Source: CAD feature listing. Evaluate the final solid. Frame: model axes, mm. Round coordinates to 2 decimals unless told otherwise and drop trailing zeros. Write each loop counter-clockwise with the first axis right and the second up, starting at its lowest first coordinate (ties: lowest second). Pieces come first, ordered by that corner, then holes. Notation, with made-up numbers: M 22,29 L 37,29 A21 cw 37,47 Z; hole C 48.25,54 d1. An arc over 180 degrees is marked long. Put each result on its own line as item: value. Start each with the question number.
```python
from build123d import *

# Parameters (mm, degrees)
SCHIZZO1_R                   = 17
SCHIZZO1_R_2                 = 2
SCHIZZO1_R_3                 = 4.5
SCHIZZO1_R_4                 = 1.5
ESTRUSIONE_ESTRUSIONE1_DEPTH = 15
M8_TAPPED_HOLE1_D            = 6.8
M8_TAPPED_HOLE1_DEPTH        = 23.75
M8_TAPPED_HOLE1_TIP          = 2.042926105


with BuildPart() as part:
    # Schizzo1 → Estrusione-Estrusione1 (new body)
    with BuildSketch(Plane.XY):
        Polygon((2, 0), (598, 0), (600, 2), (600, 98), (598, 100), (2, 100), (0, 98), (0, 2), align=None)
        with Locations((300, 38)):
            Circle(SCHIZZO1_R, mode=Mode.SUBTRACT)
        with Locations(Location((314.849242405, 52.849242405, 0), (0, 0, 180))):
            Circle(SCHIZZO1_R_2, mode=Mode.SUBTRACT)
        with Locations(Location((110, 40, 0), (0, 0, 180))):
            Circle(SCHIZZO1_R_3, mode=Mode.SUBTRACT)
        with Locations((314.849242405, 23.150757595)):
            Circle(SCHIZZO1_R_2, mode=Mode.SUBTRACT)
        with Locations(Location((285.150757595, 23.150757595, 0), (0, 0, 180))):
            Circle(SCHIZZO1_R_2, mode=Mode.SUBTRACT)
        with Locations(Location((110, 80, 0), (0, 0, 180))):
            Circle(SCHIZZO1_R_3, mode=Mode.SUBTRACT)
        with Locations(Location((536, 40, 0), (0, 0, 180))):
            Circle(SCHIZZO1_R_3, mode=Mode.SUBTRACT)
        with Locations((64, 40)):
            Circle(SCHIZZO1_R_3, mode=Mode.SUBTRACT)
        with Locations((64, 80)):
            Circle(SCHIZZO1_R_3, mode=Mode.SUBTRACT)
        with Locations((490, 40)):
            Circle(SCHIZZO1_R_3, mode=Mode.SUBTRACT)
        with Locations((15, 30)):
            Circle(SCHIZZO1_R_4, mode=Mode.SUBTRACT)
        with Locations(Location((585, 30, 0), (0, 0, 180))):
            Circle(SCHIZZO1_R_4, mode=Mode.SUBTRACT)
        with Locations((285.150757595, 52.849242405)):
            Circle(SCHIZZO1_R_2, mode=Mode.SUBTRACT)
        with Locations((490, 80)):
            Circle(SCHIZZO1_R_3, mode=Mode.SUBTRACT)
        with Locations(Location((536, 80, 0), (0, 0, 180))):
            Circle(SCHIZZO1_R_3, mode=Mode.SUBTRACT)
        with Locations((585, 70)):
            Circle(SCHIZZO1_R_4, mode=Mode.SUBTRACT)
        with Locations(Location((15, 70, 0), (0, 0, 180))):
            Circle(SCHIZZO1_R_4, mode=Mode.SUBTRACT)
    extrude(amount=-ESTRUSIONE_ESTRUSIONE1_DEPTH)

    # M8 Tapped Hole1
    with Locations(Plane(origin=(30, 0, -7.5), x_dir=(0, 0, -1), z_dir=(0, -1, 0))):
        with Locations((0, 0), (0, 540)):
            Hole(M8_TAPPED_HOLE1_D / 2, depth=M8_TAPPED_HOLE1_DEPTH)
            with Locations((0, 0, -(M8_TAPPED_HOLE1_DEPTH + M8_TAPPED_HOLE1_TIP / 2))):  # 118° drill point
                Cone(0, M8_TAPPED_HOLE1_D / 2, M8_TAPPED_HOLE1_TIP, mode=Mode.SUBTRACT)


solid = part.part
```
(1) Pull-direction query (Y, two-part tool) for faces 1 (the flat face through (296, 0, -7)), 2 (the flat face through (600, 49, -7)), 3 (the cylindrical face through (315.704, 31.489, -7.395)); classes: +Y half, -Y half, draft (parallel to the pull), parting line (faces both ways), or undercut.
(2) Section query A-A (x = 300). Return loops of the section in (y, z), and give its area (3 significant figures).
(3) Contact query for flat-ended pins moving along their axis: P1, Ø7, axis at x = 110, y = 80, coming from the +Z side; P2, Ø5, axis at x = 130, z = -10, coming from the -Y side. Output: stop coordinate, or through.
(4) Ray query, line 1 along X through (y, z) = (14.5, -7.5); line 2 along Y through (x, z) = (63, -14); line 3 along Y through (x, z) = (15, -6). Return the intervals inside material, ascending.
Entries:
1. face 1: -Y half
1. face 2: draft
1. face 3: undercut
2. outline: M 0,-15 L 21,-15 L 21,0 L 0,0 Z; M 55,-15 L 100,-15 L 100,0 L 55,0 Z
2. area: 990 mm2
3. P1: through
3. P2: y = 0
4. line 1: 0 to 26.6, 33.4 to 566.6, 573.4 to 600
4. line 2: 0 to 35.61, 44.39 to 75.61, 84.39 to 100
4. line 3: 0 to 28.5, 31.5 to 68.5, 71.5 to 100
